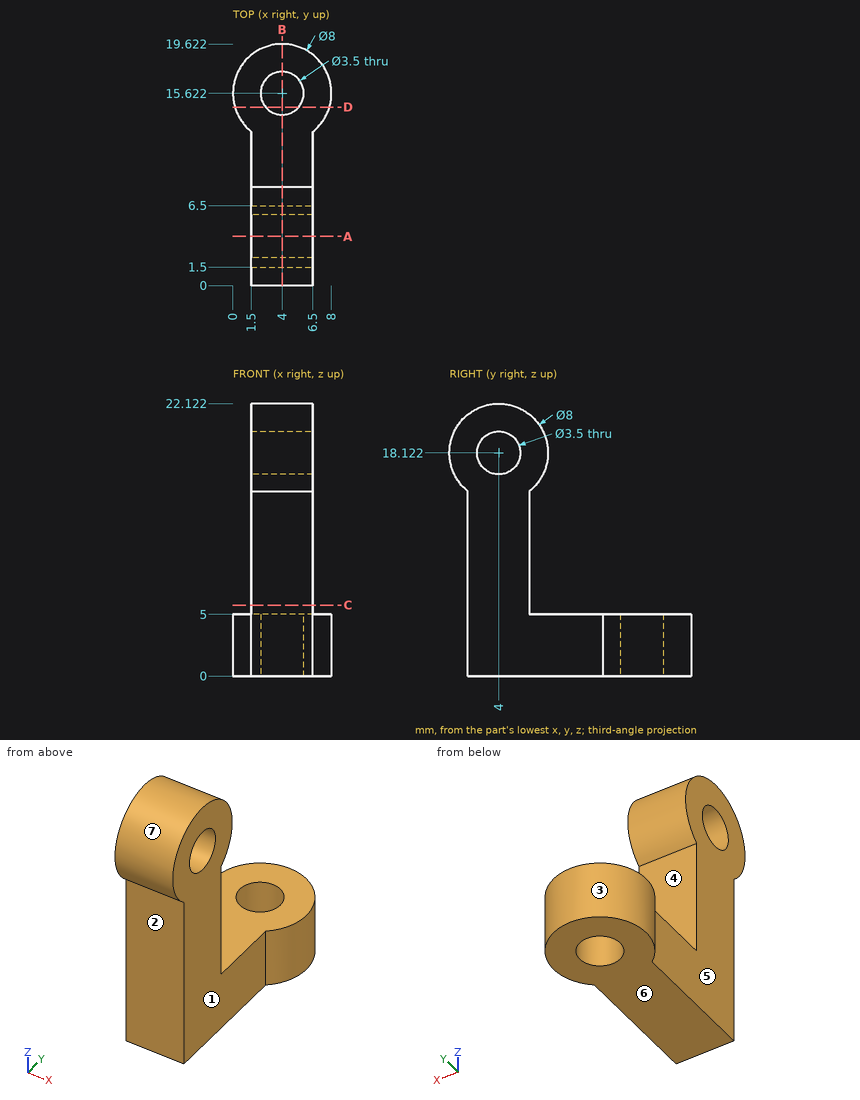
For this review, use the dimensioned drawing (mm, ordinates from the lowest corner) and the shaded views. A direction names the side the tool comes from. Give positions to 0.01 mm unless a question says otherwise; leave off trailing zeros. Write each loop counter-clockwise with the first axis right and the second up, starting at its lowest first coordinate (ties: lowest second). Pieces come first, ordered by that corner, then holes. Notation, with made-up numbers: M 8.25,62 L 16.25,62 A31 cw 16.25,92 Z; hole C -35,45.25 d8. An arc over 180 degrees is marked long. Write item = value, one per line. Start each with the question number.
Q1. We need section C-C (z = 5.75). State the section outline as (x, y) points.
Q2. For line 1 (Z direction, x = 2.65, y = 4); line 2 (Y direction, x = 4, z = 1.6); line 3 (X direction, y = 2.25, z = 5.25), list the stretches that pass through material, from the lowest coordinate up.
Q3. Mouldability with a two-part tool opening along Z and no side actions: class the marked faces 5, 6 and 7 as released by +Z, released by -Z, zero draft, split by the parting line, or undercut.
Q4. We need section A-A (y = 4). State the section outline as (x, z) points.
Q5. We need section D-D (y = 14.5). State the section outline as (x, z) points.
Q6. Clearance check with flat-ended pins moving along their axes: pin 1 (2.5 mm diameter, centred on x = 3.5, y = 16, fed in from +Z); pin 2 (1.5 mm diameter, centred on x = 3, z = 12, fed in from +Y); pin 3 (3 mm diameter, centred on x = 4.5, z = 19, fed in from +Y). State where each tip first meets the part, or that it passes through.
Q7. We need section B-B (x = 4). State the section outline as (y, z) points.
Q8. Machinability: for the marked faces 1, 2, 3 and 4, which of the approach directions +Z, -Z, +X, -X, +Y, -Y give a long, thin tool a straight path to every point of the face, cutting with its end or side? Answer none if there is none.
Result set:
q1.outline = M 1.5,1.5 L 6.5,1.5 L 6.5,6.5 L 1.5,6.5 Z
q2.line_1 = 0 to 16.37, 19.87 to 22.12
q2.line_2 = 1.5 to 13.87, 17.37 to 19.62
q2.line_3 = 1.5 to 6.5
q3.face_5 = zero draft
q3.face_6 = released by -Z
q3.face_7 = undercut
q4.outline = M 1.5,0 L 6.5,0 L 6.5,16.37 L 1.5,16.37 Z; M 1.5,19.87 L 6.5,19.87 L 6.5,22.12 L 1.5,22.12 Z
q5.outline = M 0.16,0 L 2.66,0 L 2.66,5 L 0.16,5 Z; M 5.34,0 L 7.84,0 L 7.84,5 L 5.34,5 Z
q6.pin_1 = 5
q6.pin_2 = 6.5
q6.pin_3 = 8
q7.outline = M 1.5,0 L 13.87,0 L 13.87,5 L 6.5,5 L 6.5,15 A4 ccw long 1.5,15 Z; M 17.37,0 L 19.62,0 L 19.62,5 L 17.37,5 Z; hole C 4,18.12 d3.5
q8.face_1 = +Z, -Z, +X, -Y
q8.face_2 = -Z, +X, -X, -Y
q8.face_3 = +Z, -Z
q8.face_4 = +X, -X, +Y
